from build123d import *

# Parameters (mm, degrees)
F0_W     = 11
F0_H     = 7
F1_DEPTH = 12.5
F3_DEPTH = 25
F4_DEPTH = 7
F5_R     = 2.172792
F6_R     = 1.2


with BuildPart() as f1:
    # F0 (on Front) → F1 (new body, symmetric)
    with BuildSketch(Plane.XZ):
        Polygon((14, -8), (14, 1), (5.5, 1), (-5.5, 1), (-14, 1), (-14, -8), align=None)
        with Locations((0, 4.5)):
            Rectangle(F0_W, F0_H)
    extrude(amount=F1_DEPTH, both=True)

    # F2 (on face) → F3 (cut)
    with BuildSketch(Plane(origin=(0, 0, -8), x_dir=(1, 0, 0), z_dir=(0, 0, -1))):
        with BuildLine():
            ThreePointArc((2.5, 8), (-1.767767, 9.767767), (0, 5.5))
            ThreePointArc((0, 5.5), (1.767767, 6.232233), (2.5, 8))
        make_face()
        with BuildLine():
            ThreePointArc((2.5, -8), (1.767767, -6.232233), (0, -5.5))
            ThreePointArc((0, -5.5), (-1.767767, -9.767767), (2.5, -8))
        make_face()
    extrude(amount=-F3_DEPTH, mode=Mode.SUBTRACT)

    # F2 (on face) → F4 (cut)
    with BuildSketch(Plane(origin=(0, 0, -8), x_dir=(1, 0, 0), z_dir=(0, 0, -1))):
        with BuildLine():
            ThreePointArc((4, 8), (-2.828427, 10.828427), (0, 4))
            ThreePointArc((0, 4), (2.828427, 5.171573), (4, 8))
        make_face()
        with BuildLine():
            ThreePointArc((2.5, 8), (1.767767, 6.232233), (0, 5.5))
            ThreePointArc((0, 5.5), (-1.767767, 9.767767), (2.5, 8))
        make_face(mode=Mode.SUBTRACT)
        with BuildLine():
            ThreePointArc((4, -8), (2.828427, -5.171573), (0, -4))
            ThreePointArc((0, -4), (-2.828427, -10.828427), (4, -8))
        make_face()
        with BuildLine():
            ThreePointArc((2.5, -8), (-1.767767, -9.767767), (0, -5.5))
            ThreePointArc((0, -5.5), (1.767767, -6.232233), (2.5, -8))
        make_face(mode=Mode.SUBTRACT)
    extrude(amount=-F4_DEPTH, mode=Mode.SUBTRACT)

    # F5
    f5_edges = [f1.edges().sort_by_distance(p)[0] for p in [
        (-14, -12.5, -3.5),
        (14, -12.5, -3.5),
        (14, 12.5, -3.5),
        (-14, 12.5, -3.5),
    ]]
    fillet(f5_edges, radius=F5_R)

    # F6
    f6_edges = [f1.edges().sort_by_distance(p)[0] for p in [
        (5.5, -12.5, 4.5),
        (-5.5, -12.5, 4.5),
        (5.5, 12.5, 4.5),
        (-5.5, 12.5, 4.5),
    ]]
    fillet(f6_edges, radius=F6_R)


solid = f1.part
Can you work these out from the model? Positions are in its coordinate system, mm. A direction names the side the tool comes from. Coordinates: 2 decimals unless noted, no trailing zeros. Order: outer loops, then holes, each group sorted by start corner. A loop starts at its lowest first (then second) coordinate and runs counter-clockwise, first axis right, second up. Notation, with made-up numbers: (7, 39.5) - (45, 39.5) arc R26 ccw to (45, 56.5) - close; hole circle Ø1 at (-31, -21). An arc over 180 degrees is marked (long way). Answer as a JSON object with one key per item and string values. Group by question number.
Q1. Imagine slicing it at D-D (x = 3.5). Please give me the cut outline in (y, z), and give its area (3 significant figures).
Q2. I need wall thicknesses on line 1 (X direction, y = 8, z = -5); line 2 (Y direction, x = 3.5, z = -2); line 3 (X direction, y = -8, z = 6.25). Which ranges of each line are inside material? Lowest first, please. Write a range as from..to.
Q3. On a 3-axis mill with a long thin cutter (end or side, diameter ignored), from which of +Z, -Z, +X, -X, +Y, -Y can I reach the whole of each face in a straight line? I mean faces 1 (the face through (-5.5, 0, 4)), 2 (the face through (-5.139, -12.158, 4.549)), 3 (the face through (5.139, 12.158, 4.549)). Say none if no direction works.
Q4. We'd pull the mould along X, two halves only. Please class faces 4 (the face through (-9, 0, 1)), 5 (the face through (-2, 10, -1)), 6 (the face through (-13.347, 11.88, -3.563)), 7 (the face through (-2, -6, -1)): +X half, -X half, draft (parallel to the pull), parting line (faces both ways), or undercut.
Q5. Imagine slicing it at C-C (y = -3.25). Please give me the cut outline in (x, z), and give its area (3 significant figures).
Q6. Imagine slicing it at B-B (y = -7.5). Please give me the cut outline in (x, z), and give its area (3 significant figures).
Q7. Will these pins go through, and if not, where does the flat tip stop? P1, Ø2.5, axis at x = -1.5, y = 8.5, coming from the -Z side; P2, Ø3, axis at x = 8.5, y = -5, coming from the +Z side; P3, Ø1.5, axis at x = -3, y = -5.5, coming from the -Z side; P4, Ø3.5, axis at y = -5.5, z = 6, coming from the +X side.
Q8. Imagine slicing it at A-A (z = -5.5). Please give me the cut outline in (x, y), and give its area (3 significant figures).
Determined:
{
 "1": {"outline": "(-12.5, -8) - (-9.94, -8) - (-9.94, -1) - (-6.06, -1) - (-6.06, -8) - (6.06, -8) - (6.06, -1) - (9.94, -1) - (9.94, -8) - (12.5, -8) - (12.5, 8) - (-12.5, 8) - close", "area": "346 mm2"},
 "2": {"line 1": "x = -14..-4, 4..14", "line 2": "y = -12.5..-9.94, -6.06..6.06, 9.94..12.5", "line 3": "x = -5.5..-2.5, 2.5..5.5"},
 "3": {"face 1": "+Z, -X, +Y, -Y", "face 2": "+Z, -X, -Y", "face 3": "+Z, +X, +Y"},
 "4": {"face 4": "draft", "face 5": "undercut", "face 6": "-X half", "face 7": "undercut"},
 "5": {"outline": "(-14, -8) - (14, -8) - (14, 1) - (5.5, 1) - (5.5, 8) - (-5.5, 8) - (-5.5, 1) - (-14, 1) - close", "area": "329 mm2"},
 "6": {"outline": "(-14, -8) - (-3.97, -8) - (-3.97, -1) - (-2.45, -1) - (-2.45, 8) - (-5.5, 8) - (-5.5, 1) - (-14, 1) - close; (2.45, -1) - (3.97, -1) - (3.97, -8) - (14, -8) - (14, 1) - (5.5, 1) - (5.5, 8) - (2.45, 8) - close", "area": "229 mm2"},
 "7": {"P1": "stops at z = -1", "P2": "stops at z = 1", "P3": "stops at z = -8", "P4": "stops at x = 5.5"},
 "8": {"outline": "(-14, -10.33) arc R2.17 ccw to (-11.83, -12.5) - (11.83, -12.5) arc R2.17 ccw to (14, -10.33) - (14, 10.33) arc R2.17 ccw to (11.83, 12.5) - (-11.83, 12.5) arc R2.17 ccw to (-14, 10.33) - close; hole circle Ø8 at (0, -8); hole circle Ø8 at (0, 8)", "area": "595 mm2"}
}
